CAD build for the part. Positions are in the model's coordinates, mm. Round coordinates to 2 decimals unless told otherwise and drop trailing zeros. Write each loop counter-clockwise with the first axis right and the second up, starting at its lowest first coordinate (ties: lowest second). Pieces come first, ordered by that corner, then holes. Notation, with made-up numbers: (-14.75, -25.5) - (18.25, -25.5) arc R25 cw to (18.25, -8.5) - close; hole circle Ø4 at (7, 25). An arc over 180 degrees is marked (long way). Answer in a Markdown table with one row per item.
```python
from build123d import *

# Parameters (mm, degrees)
SKETCH7_R   = 7.34
SKETCH7_R_2 = 6.34


with BuildPart() as part:
    # Sweep-Thin1: sweep along a path in Sketch1
    with BuildLine(Plane(origin=(0, 0, 0), x_dir=(1, 0, 0), z_dir=(0, 1, 0))) as sweep_thin1_path:
        Line((-186.112466625, 25.587240645), (-186.112466625, -94.412759355))
        Line((-186.112466625, -94.412759355), (-213.584309415, -543.573418645))
        ThreePointArc((-213.584309415, -543.573418645), (-219.843345577, -556.919867252), (-233.547005384, -562.352447854))
        Line((-233.547005384, -562.352447854), (-240.047005384, -562.352447854))
        ThreePointArc((-240.047005384, -562.352447854), (-253.482034226, -556.787476697), (-259.047005384, -543.352447854))
    # Sketch7 → Sweep-Thin1 (sweep)
    with BuildSketch(Plane(origin=(-259.047005384, 0, 543.352447854), x_dir=(-1, 0, 0), z_dir=(0, 0, -1))):
        Circle(SKETCH7_R)
        Circle(SKETCH7_R_2, mode=Mode.SUBTRACT)
    sweep(path=sweep_thin1_path.line, transition=Transition.RIGHT)


solid = part.part
```
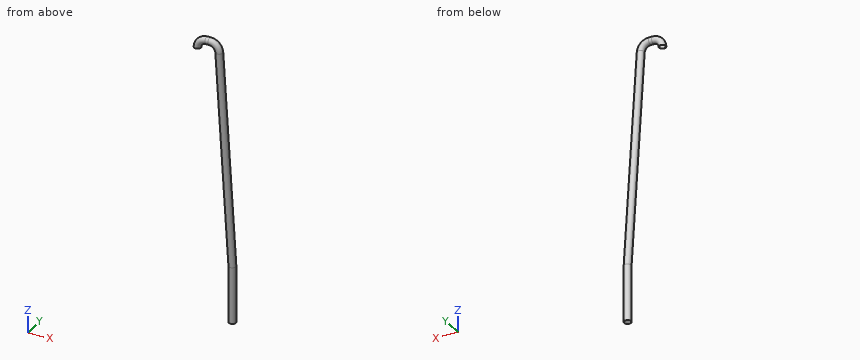
Q1. Saw through at A-A on y = -3.5. List the corners of the cut face in (x, z), then the cut area to 3 significant figures.
Computed:
| item | result |
|---|---|
| outline | (-265.5, 543.35) - (-264.33, 543.35) arc R24.29 cw to (-240.05, 567.64) - (-233.55, 567.64) arc R25.29 cw to (-208.31, 543.9) - (-180.83, 94.57) - (-180.83, -25.59) - (-179.66, -25.59) - (-179.66, 94.61) - (-207.14, 543.97) arc R26.45 ccw to (-233.55, 568.8) - (-240.05, 568.8) arc R25.45 ccw to start; (-253.76, 543.35) - (-252.6, 543.35) arc R12.55 cw to (-240.05, 555.9) - (-233.55, 555.9) arc R13.55 cw to (-220.02, 543.18) - (-192.56, 94.22) - (-192.56, -25.59) - (-191.4, -25.59) - (-191.4, 94.25) - (-218.86, 543.25) arc R14.71 ccw to (-233.55, 557.07) - (-240.05, 557.07) arc R13.71 ccw to start |
| area | 1,480 mm2 |
Q2. Drill centre lines: line 1 (Z direction, x = -236, y = 0); line 2 (X direction, y = -5.75, z = 279); line 3 (X direction, y = 4.75, z = 261.5). Where is each one in solid material? Low to high.
Computed:
| item | result |
|---|---|
| line 1 | z = 555.01 to 556.01, 568.69 to 569.69 |
| line 2 | x = -201.97 to -200.08, -194.73 to -192.83 |
| line 3 | x = -201.94 to -200.54, -192.12 to -190.73 |
Q3. Flat gauge pins, fed straight in: pin 1 (1 mm diameter, centred on x = -241, y = 1.5, fed in from -Z); pin 2 (6 mm diameter, centred on x = -256.5, y = -0.5, fed in from +Z); pin 3 (2 mm diameter, centred on y = -2, z = 241.5, fed in from +X); pin 4 (12 mm diameter, centred on x = -189.5, z = 458.5, fed in from -Y). Where does each tip first touch, or does it go through?
Computed:
| item | result |
|---|---|
| pin 1 | stops at z = 555.03 |
| pin 2 | stops at z = 565.99 |
| pin 3 | stops at x = -187.81 |
| pin 4 | passes through |
